Can you work these out from the model? Positions are in its coordinate system, mm. A direction names the side the tool comes from. Coordinates: 2 decimals unless noted, no trailing zeros. Loops run counter-clockwise (first coordinate to the right, second up) from the corner with the lowest first, then second, coordinate; pieces in that order, holes last. Notation, with made-up numbers: (-36, 52) - (16, 52) arc R38 cw to (16, 91) - close; hole circle Ø1 at (12.5, 83). An arc over 180 degrees is marked (long way). Put each result on its own line as item: value. Start each with the question number.
Autodesk Inventor part; units mm, degrees
ref_plane "Start plane" through (0, 0, 0) normal (0, 0, 1) x (1, 0, 0)
ref_plane "End plane" through (0, 0, 1140) normal (0, 0, 1) x (1, 0, 0)
ref_plane "Work Plane4" through (-85, 0, 1140) normal (0, 0, 1) x (1, 0, 0)
ref_plane "Start plane" through (0, 0, 0) normal (0, 0, 1) x (1, 0, 0)
ref_plane "End plane" through (0, 0, 1140) normal (0, 0, 1) x (1, 0, 0)
sketch "Sketch2" plane through (0, 0, 0) normal (0, 0, 1) x (1, 0, 0)
  line L0 (-55, 100.8) -> (-14.95, 100.8)
  line L1 (-55, 110) -> (-55, 100.8)
  line L2 (55, 110) -> (-55, 110)
  line L3 (55, 100.8) -> (55, 110)
  line L4 (14.95, 100.8) -> (55, 100.8)
  line L5 (2.95, -88.8) -> (2.95, 88.8)
  line L6 (55, -100.8) -> (14.95, -100.8)
  line L7 (55, -110) -> (55, -100.8)
  line L8 (-55, -100.8) -> (-55, -110)
  line L9 (-14.95, -100.8) -> (-55, -100.8)
  line L10 (-2.95, 88.8) -> (-2.95, -88.8)
  line L11 (0, -154) -> (0, 154) construction
  line L12 (-2.95, -100.8) -> (2.95, -100.8) construction
  arc A0 (-14.95, -100.8) -> (-2.95, -88.8) centre (-14.95, -88.8) ccw
  arc A1 (-2.95, 88.8) -> (-14.95, 100.8) centre (-14.95, 88.8) ccw
  arc A2 (14.95, 100.8) -> (2.95, 88.8) centre (14.95, 88.8) ccw
  arc A3 (2.95, -88.8) -> (14.95, -100.8) centre (14.95, -88.8) ccw
  line L13 (-77, 0) -> (77, 0) construction
  line L14 (-55, -110) -> (55, -110)
  point P0 (-2.95, 100.8)
  point P1 (2.95, 100.8)
  point P2 (0, 0)
  point P3 (0, -100.8)
  point P4 (0, 0)
  dimension "d1" = 220
  dimension "d3" = 9.2
  dimension "d5" = 5.9
  dimension "d7" = 110
  dimension "d13" = 12
  dimension "d14" = 110
  dimension "d15" = 55
extrude "Body" add sketch "Sketch2" along normal up to surface (1140 mm away) from surface at 0
sketch "Sketch3" plane through (0, 0, 0) normal (0, 0, 1) x (1, 0, 0)
  line L0 (0, 0) -> (10, 0)
ref_plane "Work Plane3" through (0, 0, 0) normal (0, -1, 0) x (1, 0, 0)
ref_plane "Work Plane4" through (-85, 0, 1140) normal (0, 0, 1) x (1, 0, 0)
split "Split1" plane through (-85, 0, 1140) removes the side toward (0, 0, 1)
sketch "Sketch4" plane through (0, 0, 0) normal (0, -1, 0) x (1, 0, 0)
  line L0 (-2, 0) -> (12, 0)
  line L1 (-2, 1140) -> (12, 1140)
  dimension "d19" = 1140
equation "\"d1\" = ParH"
equation "\"d3\" = t2"
equation "\"d7\" = b"
equation "\"d13\" = R1"
equation "\"d14\" = 0.5 * d1"
equation "\"d15\" = 0.5 * d7"
equation "\"d8\" = G_L"
equation "\"b\" = 110"
equation "\"ParH\" = 220"
equation "\"R1\" = 12"
equation "\"G_L\" = d19"
equation "\"t1\" = 5.9"
equation "\"t2\" = 9.2"
equation "\"G_OFFSET_START\" = 0"
properties part number "DIN 1025 - IPE 220-1140" material "Steel, Mild"
Q1. I want a section at B-B on z = 625. List the corners of the cut face in (x, y) for me, and give its area (3 significant figures).
Q2. Please list where these lines run through material, in increasing order: line 1 along Y through (x, z) = (-16.5, 242); line 2 along X through (y, z) = (-66, 1082); line 3 along Y through (x, z) = (-5.5, 670.5). Write a range as [from, to].
Q3. I want a section at A-A on x = 29.5. List the corners of the cut face in (y, z) for me.
Q4. On a 3-axis mill with a long thin cutter (end or side, diameter ignored), from which of +Z, -Z, +X, -X, +Y, -Y can I reach the whole of each face in a straight line? I mean faces 1 (the flat face through (35, 100.8, 562)), 2 (the flat face through (-35, 100.8, 562)), 3 (the flat face through (0, 1, 0)). Say none if no direction works.
Q5. Will these pins go through, and if not, where does the flat tip stop? pin 1 (12 mm diameter, centred on y = 39.5, z = 959, fed in from -X); pin 2 (1 mm diameter, centred on y = 14.5, z = 465.5, fed in from +X).
Q6. We'd pull the mould along Y, two halves only. Please class faces 4 (the flat face through (-1, -110, 562)), 5 (the flat face through (1, 110, 562)), 6 (the flat face through (-2.95, 1, 562)), 7 (the flat face through (0, 1, 1140)): released by +Y, released by -Y, zero draft, split by the parting line, or undercut.
Q7. I want a section at C-C on y = -71. List the corners of the cut face in (x, z) for me, and give its area (3 significant figures).
Calculated:
1. outline: (-55, -110) - (55, -110) - (55, -100.8) - (14.95, -100.8) arc R12 cw to (2.95, -88.8) - (2.95, 88.8) arc R12 cw to (14.95, 100.8) - (55, 100.8) - (55, 110) - (-55, 110) - (-55, 100.8) - (-14.95, 100.8) arc R12 cw to (-2.95, 88.8) - (-2.95, -88.8) arc R12 cw to (-14.95, -100.8) - (-55, -100.8) - close
1. area: 3,340 mm2
2. line 1: [-110, -100.8], [100.8, 110]
2. line 2: [-2.95, 2.95]
2. line 3: [-110, -96.2], [96.2, 110]
3. outline: (-110, 0) - (-100.8, 0) - (-100.8, 1140) - (-110, 1140) - close; (100.8, 0) - (110, 0) - (110, 1140) - (100.8, 1140) - close
4. face 1: +Z, -Z, +X
4. face 2: +Z, -Z, -X
4. face 3: -Z, +X, -X, +Y, -Y
5. pin 1: x = -2.95
5. pin 2: x = 2.95
6. face 4: released by -Y
6. face 5: released by +Y
6. face 6: undercut
6. face 7: zero draft
7. outline: (-2.95, 0) - (2.95, 0) - (2.95, 1140) - (-2.95, 1140) - close
7. area: 6,730 mm2
